```python
from build123d import *

# Parameters (mm, degrees)
SKETCH1_R           = 3.175
SKETCH1_W           = 7.9375
SKETCH1_H           = 7.9375
BOSS_EXTRUDE1_DEPTH = 1.27


with BuildPart() as part:
    # Sketch1 → Boss-Extrude1 (new body)
    with BuildSketch(Plane(origin=(0, 0, 0), x_dir=(1, 0, 0), z_dir=(0, 1, 0))):
        Polygon((-20.6375, 5.08), (-5.08, 5.08), (-5.08, 20.6375), (5.08, 20.6375), (5.08, 5.08), (20.6375, 5.08), (20.6375, -5.08), (5.08, -5.08), (5.08, -20.6375), (-5.08, -20.6375), (-5.08, -5.08), (-20.6375, -5.08), align=None)
        with Locations(Location((0, 0, 0), (0, 0, 270))):
            Circle(SKETCH1_R, mode=Mode.SUBTRACT)
        with Locations((8.89, 0)):
            Rectangle(SKETCH1_W, SKETCH1_H, mode=Mode.SUBTRACT)
        with Locations((-8.89, 0)):
            Rectangle(SKETCH1_W, SKETCH1_H, mode=Mode.SUBTRACT)
    extrude(amount=BOSS_EXTRUDE1_DEPTH)


solid = part.part
```
Verification items for the finished model (mm, model axes). A direction names the side the tool comes from. Give positions to 0.01 mm unless a question says otherwise; leave off trailing zeros. Order: outer loops, then holes, each group sorted by start corner. A loop starts at its lowest first (then second) coordinate and runs counter-clockwise, first axis right, second up. Notation, with made-up numbers: M 25.25,47.5 L 37.25,47.5 A24 ccw 37.25,75.5 Z; hole C 38.25,29.5 d3. An arc over 180 degrees is marked long. Answer in a Markdown table with one row per item. Add a question column.
Item 1: Mould release check, pull along X, two halves, no side actions. Record for faces 6 (the flat face through (-5.08, 1, 13)), 7 (the flat face through (13, 1, -5.08)), 8 (the flat face through (12.859, 1, 0)): released by +X, released by -X, zero draft, split by the parting line, or undercut.
Item 2: Tool access check on faces 1 (the flat face through (20.638, 1, 0)), 2 (the flat face through (-4.921, 1, 0)), 3 (the flat face through (13, 1, 5.08)), 4 (the flat face through (-13, 1, 5.08)), 5 (the flat face through (-5.08, 1, -13)). Record the directions out of +Z, -Z, +X, -X, +Y, -Y that give a thin tool (end or side, any length) a straight path to the whole face; none if there is none.
Item 3: Section check D-D, the plane x = 0. Enter the section's corners in (y, z) (1 decimal).
Item 4: Section check C-C, the plane y = 0.3. State how many separate pieces and enclosed holes the cut face has, and give its area (3 significant figures).
Item 5: Gauge pin test, flat end, axial feed: pin 1 (0.6 mm diameter, centred on x = -11, y = 0.5, fed in from -Z). Record the tip position at first contact, or that the pin passes through.
Item 6: Scan lines: probe 1 along X at (y, z) = (0.6, 0) (1 decimal); probe 2 along Z at (x, y) = (9, 0.6); probe 3 along Z at (x, y) = (-16.5, 0.9). Record each from-to range of solid material in increasing order. Write a range as from..to.
Item 7: Section check B-B, the plane z = 0. Enter the section's corners in (x, y) (1 decimal).
Item 8: Section check A-A, the plane x = -6.5. Enter the section's corners in (y, z), and give its area (3 significant figures).
Filled sheet:
| question | item | result |
|---|---|---|
| 1 | face 6 | released by -X |
| 1 | face 7 | zero draft |
| 1 | face 8 | undercut |
| 2 | face 1 | +Z, -Z, +X, +Y, -Y |
| 2 | face 2 | +Y, -Y |
| 2 | face 3 | +Z, +X, +Y, -Y |
| 2 | face 4 | +Z, -X, +Y, -Y |
| 2 | face 5 | -Z, -X, +Y, -Y |
| 3 | outline | M 0,-20.6 L 1.3,-20.6 L 1.3,-3.2 L 0,-3.2 Z; M 0,3.2 L 1.3,3.2 L 1.3,20.6 L 0,20.6 Z |
| 4 | separate pieces | 1 |
| 4 | enclosed holes | 3 |
| 4 | area | 578 mm^2 |
| 5 | pin 1 | stops at z = -5.08 |
| 6 | probe 1 | x = -20.6..-12.9, -4.9..-3.2, 3.2..4.9, 12.9..20.6 |
| 6 | probe 2 | z = -5.08..-3.97, 3.97..5.08 |
| 6 | probe 3 | z = -5.08..5.08 |
| 7 | outline | M -20.6,0 L -12.9,0 L -12.9,1.3 L -20.6,1.3 Z; M -4.9,0 L -3.2,0 L -3.2,1.3 L -4.9,1.3 Z; M 3.2,0 L 4.9,0 L 4.9,1.3 L 3.2,1.3 Z; M 12.9,0 L 20.6,0 L 20.6,1.3 L 12.9,1.3 Z |
| 8 | outline | M 0,-5.08 L 1.27,-5.08 L 1.27,-3.97 L 0,-3.97 Z; M 0,3.97 L 1.27,3.97 L 1.27,5.08 L 0,5.08 Z |
| 8 | area | 2.82 mm^2 |
